Model file for the job. Use its own axes, mm. A direction names the side the tool comes from. Coordinates: 2 decimals unless noted, no trailing zeros. Order: outer loops, then holes, each group sorted by start corner. A loop starts at its lowest first (then second) coordinate and runs counter-clockwise, first axis right, second up. Notation, with made-up numbers: M 19,-39 L 64,-39 A7 cw 64,-34 Z; hole C 24.5,73 d10. An arc over 180 degrees is marked long. Return JSON: item names as keys, results as strings.
```python
from build123d import *

# Parameters (mm, degrees)
COVER_START       = -397
COVER_DEPTH       = 437.1
RAIL_START        = -400
RAIL_FLANGE_DEPTH = 443.1


with BuildPart() as part:
    # Sketch1 → Cover (new body)
    with BuildSketch(Plane.XY.offset(COVER_START)):
        with BuildLine():
            Line((-193.711902706, 287.049997823), (-287.049997823, 193.711902706))
            Line((-287.049997823, 193.711902706), (-305.717616846, 212.379521729))
            ThreePointArc((-305.717616846, 212.379521729), (-312.044110372, 227.653028203), (-305.717616846, 242.926534677))
            Line((-305.717616846, 242.926534677), (-242.926534677, 305.717616846))
            ThreePointArc((-242.926534677, 305.717616846), (-227.653028203, 312.044110372), (-212.379521729, 305.717616846))
            Line((-212.379521729, 305.717616846), (-193.711902706, 287.049997823))
        make_face()
    extrude(amount=COVER_DEPTH)

    # Sketch2 → Rail Flange (add)
    with BuildSketch(Plane.XY.offset(RAIL_START)):
        Polygon((-191.590582362, 289.171318166), (-289.171318166, 191.590582362), (-293.413958853, 195.83322305), (-195.83322305, 293.413958853), align=None)
    extrude(amount=RAIL_FLANGE_DEPTH)


solid = part.part
```
Item 1: Pull direction Y, two halves, no side cores. Call faces 1 (the flat face through (-254, 256, 40.1)), 2 (the flat face through (-239.7, 241.06, -181.55)), 3 (the flat face through (-291.835, 197.413, -179.484)): +Y half, -Y half, draft (parallel to the pull), parting line (faces both ways), or undercut.
Check result:
{"face 1": "draft", "face 2": "-Y half", "face 3": "undercut"}
Item 2: Drop flat-ended pins along their axis: pin 1 Ø12 at (y, z) = (289.5, -161) entering from -X; pin 2 Ø1.5 at (y, z) = (207.5, -228) entering from +X; pin 3 Ø12 at (y, z) = (248.5, -115.5) entering from +X. Give the stop position or say it passes through.
Check result:
{"pin 1": "stops at x = -265.14", "pin 2": "stops at x = -272.51", "pin 3": "stops at x = -226.26"}
Item 3: 3-axis set-ups, long thin cutter, end or side, ignore diameter. For faces 4 (the cylindrical face through (-227.891, 312.043, -181.51)), 5 (the flat face through (-254, 256, -397)): which of +Z, -Z, +X, -X, +Y, -Y reach the whole face in a straight line?
Check result:
{"face 4": "+Z, -Z, +Y", "face 5": "-Z, -X, +Y"}
Item 4: Saw through at B-B (x = -235). Write the cut outline in (y, z), and give its area (3 significant figures).
Check result:
{"outline": "M 245.76,-400 L 254.25,-400 L 254.25,-397 L 310.76,-397 L 310.76,40.1 L 254.25,40.1 L 254.25,43.1 L 245.76,43.1 Z", "area": "28,500 mm2"}
Item 5: Saw through at A-A (z = -127). Write the cut outline in (x, y).
Check result:
{"outline": "M -305.72,212.38 L -291.29,197.95 L -293.41,195.83 L -289.17,191.59 L -191.59,289.17 L -195.83,293.41 L -197.95,291.29 L -212.38,305.72 A21.6 ccw -242.93,305.72 L -305.72,242.93 A21.6 ccw Z"}
Item 6: Saw through at C-C (y = 283.5). Write the cut outline in (x, z).
Check result:
{"outline": "M -265.14,-397 L -205.75,-397 L -205.75,-400 L -197.26,-400 L -197.26,43.1 L -205.75,43.1 L -205.75,40.1 L -265.14,40.1 Z"}
Item 7: Wall check: line 1 (Z direction, x = -294, y = 215); line 2 (Y direction, x = -208.5, z = -257); line 3 (Y direction, x = -236, z = -138). Give the ranges that are in metal, low to high.
Check result:
{"line 1": "z = -397 to 40.1", "line 2": "y = 272.26 to 301.84", "line 3": "y = 244.76 to 310.37"}
